Autodesk Inventor part; units mm, degrees
ref_plane "Work Plane2" through (-24.0216, -23.1431, 0) normal (0, 0, 1) x (1, 0, 0)
ref_plane "YZ Plane" through (0, 0, 0) normal (1, 0, 0) x (0, 1, 0)
ref_plane "XZ Plane" through (0, 0, 0) normal (0, 1, 0) x (-1, 0, 0)
ref_plane "Work Plane1" through (0, 0, 0) normal (0, 0, 1) x (1, 0, 0)
sketch "Sketch3" plane through (0, 0, 0) normal (0, 0, 1) x (1, 0, 0)
  line L0 (-22.0216, 21.1569) -> (-22.0216, -21.1431)
  line L1 (-0.0216, 21.1569) -> (-22.0216, 21.1569)
  line L2 (-0.0216, 23.1569) -> (-0.0216, 21.1569)
  line L3 (-0.0216, 23.1569) -> (-22.0216, 23.1569)
  arc A0 (-22.0216, 23.1569) -> (-24.0216, 21.1569) centre (-22.0216, 21.1569) ccw
  line L4 (-24.0216, -21.1431) -> (-24.0216, 21.1569)
  arc A1 (-24.0216, -21.1431) -> (-22.0216, -23.1431) centre (-22.0216, -21.1431) ccw
  line L5 (-22.0216, -23.1431) -> (-0.0216, -23.1431)
  line L6 (-0.0216, -21.1431) -> (-0.0216, -23.1431)
  line L7 (-22.0216, -21.1431) -> (-0.0216, -21.1431)
  line L8 (0.2784, 23.1569) -> (0.2784, 21.1569)
  line L9 (12.9784, 21.1569) -> (0.2784, 21.1569)
  line L10 (21.9784, 12.1569) -> (12.9784, 21.1569)
  line L11 (21.9784, -12.1431) -> (21.9784, 12.1569)
  line L12 (12.9784, -21.1431) -> (21.9784, -12.1431)
  line L13 (0.2784, -21.1431) -> (12.9784, -21.1431)
  line L14 (0.2784, -21.1431) -> (0.2784, -23.1431)
  line L15 (23.9784, -23.1431) -> (0.2784, -23.1431)
  line L16 (23.9784, 23.1569) -> (23.9784, -23.1431)
  line L17 (0.2784, 23.1569) -> (23.9784, 23.1569)
  line L18 (0.2784, 21.1569) -> (-0.0216, 21.1569)
  line L19 (-0.0216, 21.1569) -> (-0.0216, 23.1569)
  line L20 (-0.0216, 23.1569) -> (0.2784, 23.1569)
  line L21 (0.2784, 23.1569) -> (0.2784, 21.1569)
  line L22 (-0.0216, -21.1431) -> (0.2784, -21.1431)
  line L23 (0.2784, -21.1431) -> (0.2784, -23.1431)
  line L24 (0.2784, -23.1431) -> (-0.0216, -23.1431)
  line L25 (-0.0216, -23.1431) -> (-0.0216, -21.1431)
  point P0 (0, 0)
extrude "Extrusion2" add sketch "Sketch3" along normal blind 25.75 contours L0 L7 L6 L5 A1 L4 A0 L3 L2 L1 | L2 L20 L8 L18 | L22 L14 L24 L6 | L8 L17 L16 L15 L14 L13 L12 L11 L10 L9
sketch "Sketch5" plane through (23.9784, -23.1431, 0) normal (1, 0, 0) x (0, 0, -1)
  circle A0 centre (-12.875, 23.1431) radius 7.5
  point P0 (0, 23.1431)
  dimension "d4" = 15
extrude "Extrusion3" cut sketch "Sketch5" against normal up to surface (2 mm away)
sketch "Sketch7" plane through (0, 0, 25.75) normal (0, 0, 1) x (1, 0, 0)
  line L0 (-22.0216, -21.1431) -> (12.9784, -21.1431)
  line L1 (-22.0216, 21.1569) -> (-22.0216, -21.1431)
  line L2 (-22.0216, -12.1431) -> (-22.0216, -21.1431)
  line L3 (-22.0216, -12.1431) -> (-13.0216, -21.1431)
  line L4 (-22.0216, -21.1431) -> (-13.0216, -21.1431)
  line L5 (-13.0216, 21.1569) -> (-22.0216, 21.1569)
  line L6 (-13.0216, 21.1569) -> (-22.0216, 12.1569)
  line L7 (-22.0216, 21.1569) -> (-22.0216, 12.1569)
  point P0 (0, 0)
ref_plane "Work Plane2" through (-24.0216, -23.1431, 0) normal (0, 0, 1) x (1, 0, 0)
extrude "Extrusion5" add sketch "Sketch7" against normal up to surface (25.75 mm away)
sketch "Sketch8" plane through (23.9784, -23.1431, 0) normal (1, 0, 0) x (0, 0, -1)
  circle A0 centre (-11.625, 39.8) radius 1.25
  circle A1 centre (-11.625, 6.5) radius 1.25
  point P0 (0, 23.1431)
extrude "Extrusion6" cut sketch "Sketch8" against normal blind 25.75
properties part number "MotorHousingBottom_split3"
Build history of the part. All positions in model axes, mm. A direction names the side the tool comes from. Coordinates: 2 decimals unless noted, no trailing zeros. Order: outer loops, then holes, each group sorted by start corner. A loop starts at its lowest first (then second) coordinate and runs counter-clockwise, first axis right, second up. Notation, with made-up numbers: (78, -7.75) - (97, -7.75) arc R35 cw to (97, 24.25) - close; hole circle Ø9 at (-8.75, 81). An arc over 180 degrees is marked (long way). Write each question's results on one line, items separated by ' | '. Start each with the question number.
Item 1: Flat gauge pin, fed straight in: pin 1 (2 mm diameter, centred on y = 16.66, z = 11.62, fed in from +X). Where does the tip first touch, or does it go through?
Item 2: Band-saw the part on B-B on y = 0. Write the cut outline in (x, z) (3 decimals).
Item 3: Wall check: probe 1 along X at (y, z) = (4, 5); probe 2 along Y at (x, z) = (9, 6.75); probe 3 along Y at (x, z) = (-18, 14). Give the ranges that are in metal, low to high. Write a range as [from, to].
Item 4: Mould opens along X. For faces 4 (the face through (0, -21.143, 13)), 5 (the face through (-23.42, -22.573, 12.695)), 6 (the face through (23.978, 5, 7)) say: released by +X, released by -X, zero draft, split by the parting line, or undercut.
Item 5: Band-saw the part on A-A on x = 4. Write the cut outline in (y, z), and give its area (3 significant figures).
Item 6: Band-saw the part on C-C on z = 22.25. Write the cut outline in (x, y).
Item 7: Band-saw the part on D-D on z = 11.5. Write the cut outline in (x, y), and give its area (3 significant figures).
Item 8: Tool access for faces 1 (the face through (18.541, 15.594, 12.695)), 2 (the face through (-5, -22, 0)), 3 (the face through (21.017, 17.896, 11.788)): list every direction of +Z, -Z, +X, -X, +Y, -Y with a clear straight run to the whole face (end or side of a thin tool).
Numbers:
1) pin 1: x = -16.52
2) outline: (-24.022, 0) - (-22.022, 0) - (-22.022, 25.75) - (-24.022, 25.75) - close; (21.978, 0) - (23.978, 0) - (23.978, 5.375) - (21.978, 5.375) - close; (21.978, 20.375) - (23.978, 20.375) - (23.978, 25.75) - (21.978, 25.75) - close
3) probe 1: [-24.02, -22.02], [21.98, 23.98] | probe 2: [-23.14, -21.14], [21.16, 23.16] | probe 3: [-23.14, -16.16], [16.18, 23.16]
4) face 4: undercut | face 5: released by -X | face 6: released by +X
5) outline: (-23.14, 0) - (-21.14, 0) - (-21.14, 25.75) - (-23.14, 25.75) - close; (21.16, 0) - (23.16, 0) - (23.16, 25.75) - (21.16, 25.75) - close | area: 103 mm^2
6) outline: (-24.02, -21.14) arc R2 ccw to (-22.02, -23.14) - (23.98, -23.14) - (23.98, 23.16) - (-22.02, 23.16) arc R2 ccw to (-24.02, 21.16) - close; hole (-22.02, -12.14) - (-13.02, -21.14) - (12.98, -21.14) - (21.98, -12.14) - (21.98, 12.16) - (12.98, 21.16) - (-13.02, 21.16) - (-22.02, 12.16) - close
7) outline: (-24.02, -21.14) arc R2 ccw to (-22.02, -23.14) - (23.98, -23.14) - (23.98, -17.89) - (16.23, -17.89) - (12.98, -21.14) - (-13.02, -21.14) - (-22.02, -12.14) - (-22.02, 12.16) - (-13.02, 21.16) - (12.98, 21.16) - (16.23, 17.9) - (23.98, 17.9) - (23.98, 23.16) - (-22.02, 23.16) arc R2 ccw to (-24.02, 21.16) - close; (18.72, -15.4) - (23.98, -15.4) - (23.98, -7.37) - (21.98, -7.37) - (21.98, -12.14) - close; (18.72, 15.41) - (21.98, 12.16) - (21.98, 7.37) - (23.98, 7.37) - (23.98, 15.41) - close | area: 460 mm^2
8) face 1: +Z, -Z | face 2: -Z, +X, -X, +Y, -Y | face 3: +X
